```python
from build123d import *

# Parameters (mm, degrees)
F3_DEPTH = 49.784
F4_R     = 19.670017
F5_DEPTH = 4.572


with BuildPart() as f1:
    # F0 (on Front) → F1 (revolve)
    with BuildSketch(Plane.XZ):
        Polygon((4.108123, 17.581305), (-1.987877, 17.581305), (-8.539953, 29.660342), (-13.619953, 29.660342), (-13.619953, 25.989784), (-11.896132, 25.989784), (-9.338465, 17.581305), (-9.338465, 0), (14.451806, 0), (14.451806, 29.21), (9.341924, 29.21), align=None)
    revolve(axis=Axis((2.55667, 0, 0), (-1, 0, 0)))

    # F2 (on face) → F3 (cut)
    with BuildSketch(Plane.YZ.offset(14.451806)):
        with BuildLine():
            Line((-2.171075, 11.435072), (-2.171075, 9.300354))
            ThreePointArc((-2.171075, 9.300354), (0, -9.5504), (2.171075, 9.300354))
            Line((2.171075, 9.300354), (2.171075, 11.435072))
            Line((2.171075, 11.435072), (-2.171075, 11.435072))
        make_face()
    extrude(amount=-F3_DEPTH, mode=Mode.SUBTRACT)

    # F4 (on face) → F5 (join)
    with BuildSketch(Plane.YZ.offset(14.451806)):
        Circle(F4_R)
        with BuildLine():
            Line((2.171075, 11.435072), (2.171075, 9.300354))
            ThreePointArc((2.171075, 9.300354), (0, -9.5504), (-2.171075, 9.300354))
            Line((-2.171075, 9.300354), (-2.171075, 11.435072))
            Line((-2.171075, 11.435072), (2.171075, 11.435072))
        make_face(mode=Mode.SUBTRACT)
    extrude(amount=F5_DEPTH)


solid = f1.part
```
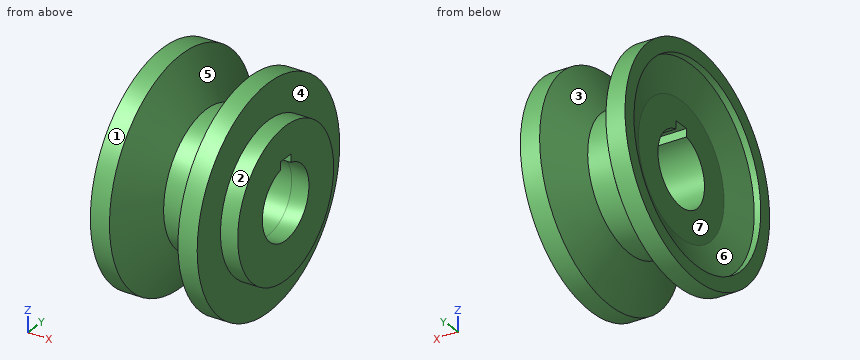
Could you check a few things on this model? Use its own coordinates, in mm. Face numbers are marked on the shaded views. A direction names the side the tool comes from. Give positions to 0.01 mm unless a question says otherwise; leave off trailing zeros. Write each loop counter-clockwise with the first axis right and the second up, starting at its lowest first coordinate (ties: lowest second). Pieces come first, ordered by that corner, then holes. Notation, with made-up numbers: (-23.75, -27) -> (-19.75, -27) arc R26 ccw to (-19.75, -13) -> close; hole circle Ø3 at (44, -29.5). An arc over 180 degrees is marked (long way). Write each question's results on one line, items separated by ' | '.
1. If we mould it in two halves opening along Y, with no side actions, what happens to the marked faces 4, 5, 6 and 7? For each: released by +Y, released by -Y, zero draft, split by the parting line, or undercut.
Check sheet entries:
face 4: zero draft | face 5: split by the parting line | face 6: undercut | face 7: undercut
2. I need wall thicknesses on L1, parallel to Y at x = 0.25, z = 0; L2, parallel to Z at x = 16, y = 0; L3, parallel to X at y = 14.5, z = -9. Which ranges of each line are inside material? Lowest first, please.
Check sheet entries:
L1: y = -17.58 to -9.55, 9.55 to 17.58 | L2: z = -19.67 to -9.55, 11.44 to 19.67 | L3: x = -9.34 to 19.02
3. I want a section at C-C, the plane x = -3.5. Write out the boundary of the cut face in (y, z).
Check sheet entries:
outline: circle Ø40.74 at (0, 0); hole (-2.17, 9.3) arc R9.55 ccw (long way) to (2.17, 9.3) -> (2.17, 11.44) -> (-2.17, 11.44) -> close
4. I want a section at A-A, the plane y = 0. Write out the boundary of the cut face in (x, z), then the cut area to 3 significant figures.
Check sheet entries:
outline: (-13.62, -29.66) -> (-8.54, -29.66) -> (-1.99, -17.58) -> (4.11, -17.58) -> (9.34, -29.21) -> (14.45, -29.21) -> (14.45, -19.67) -> (19.02, -19.67) -> (19.02, -9.55) -> (-9.34, -9.55) -> (-9.34, -17.58) -> (-11.9, -25.99) -> (-13.62, -25.99) -> close; (-13.62, 25.99) -> (-11.9, 25.99) -> (-9.34, 17.58) -> (-9.34, 11.44) -> (19.02, 11.44) -> (19.02, 19.67) -> (14.45, 19.67) -> (14.45, 29.21) -> (9.34, 29.21) -> (4.11, 17.58) -> (-1.99, 17.58) -> (-8.54, 29.66) -> (-13.62, 29.66) -> close | area: 752 mm²
5. On a 3-axis mill with a long thin cutter (end or side, diameter ignored), from which of +Z, -Z, +X, -X, +Y, -Y can I reach the whole of each face in a straight line? I mean the marked faces 1, 2 and 3. Say none if no direction works.
Check sheet entries:
face 1: +X, -X | face 2: +X | face 3: none
6. Will these pins go through, and if not, where does the flat tip stop? pin 1 Ø5 at (x, z) = (8.5, 10) entering from -Y; pin 2 Ø3 at (x, y) = (4, -1) entering from +Z; pin 3 Ø3.5 at (x, y) = (11.5, -1) entering from -Z.
Check sheet entries:
pin 1: stops at y = -28.19 | pin 2: stops at z = 20.65 | pin 3: stops at z = -29.21
7. I want a section at B-B, the plane z = 0. Write out the boundary of the cut face in (x, y).
Check sheet entries:
outline: (-13.62, -29.66) -> (-8.54, -29.66) -> (-1.99, -17.58) -> (4.11, -17.58) -> (9.34, -29.21) -> (14.45, -29.21) -> (14.45, -19.67) -> (19.02, -19.67) -> (19.02, -9.55) -> (-9.34, -9.55) -> (-9.34, -17.58) -> (-11.9, -25.99) -> (-13.62, -25.99) -> close; (-13.62, 25.99) -> (-11.9, 25.99) -> (-9.34, 17.58) -> (-9.34, 9.55) -> (19.02, 9.55) -> (19.02, 19.67) -> (14.45, 19.67) -> (14.45, 29.21) -> (9.34, 29.21) -> (4.11, 17.58) -> (-1.99, 17.58) -> (-8.54, 29.66) -> (-13.62, 29.66) -> close
